Check sheet for the drawn part. Datum: minimum x, y, z corner. Units: mm. A direction names the side the tool comes from. Give positions to 0.01 mm unless a question says otherwise; leave off trailing zeros. Order: outer loops, then holes, each group sorted by start corner. A loop starts at its lowest first (then second) coordinate and runs counter-clockwise, first axis right, second up. Notation, with made-up numbers: (88, 51) - (96, 51) arc R24 cw to (96, 62) - close; hole circle Ø7 at (-12, 77.25). An arc over 180 degrees is marked (long way). Answer as a JSON object with one key per item and string values. Group by question number.
(1) Section check D-D (y = 15). Record the boundary of the cut face in (x, z).
(2) Section check C-C (z = 12). Record the boundary of the cut face in (x, y), then the cut area to 3 significant figures.
(3) Access from +Z, -Z, +X, -X, +Y, -Y to the whole of each face (thin tool, end or side, straight path). Record for the marked faces 5 and 6.
(4) Section check A-A (x = 21). Record the boundary of the cut face in (y, z).
(5) Depth check by flat-ended pin: pin 1 Ø6 at (x, z) = (27.5, 10.5) entering from +Y; pin 2 Ø1 at (x, z) = (18, 16.5) entering from -Y; pin 3 Ø13 at (x, y) = (18.5, 22.5) entering from -Z; pin 4 Ø10 at (x, z) = (20.5, 25) entering from -Y. Enter the tip coordinate at first touch or a pass-through.
(6) Mould release check, pull along Z, two halves, no side actions. Record for the marked faces 1, 2, 3 and 4: +Z half, -Z half, draft (parallel to the pull), parting line (faces both ways), or undercut.
(7) Section check B-B (z = 32). Record the boundary of the cut face in (x, y), then the cut area to 3 significant figures.
(8) Thickness scan on line 1 (Y direction, x = 29, z = 33.5); line 2 (X direction, y = 32.5, z = 8); line 3 (Y direction, x = 13, z = 31) (3 decimals). Record the ranges inside material, lowest first.
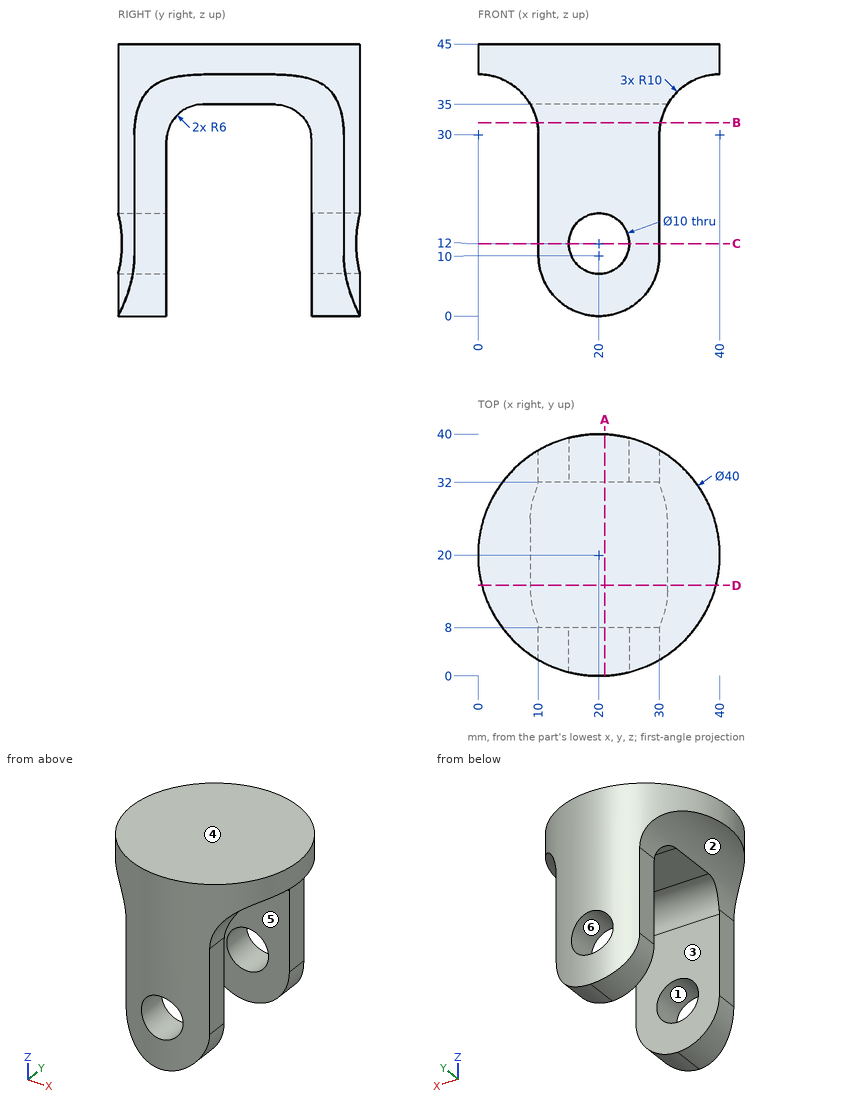
Solutions:
{
 "1": {"outline": "(0.64, 39.98) arc R10 cw to (8.66, 35) - (31.34, 35) arc R10 cw to (39.36, 39.98) - (39.36, 45) - (0.64, 45) - close"},
 "2": {"outline": "(10, 2.68) arc R20 ccw to (15, 0.64) - (15, 8) - (10, 8) - close; (10, 32) - (15, 32) - (15, 39.36) arc R20 ccw to (10, 37.32) - close; (25, 0.64) arc R20 ccw to (30, 2.68) - (30, 8) - (25, 8) - close; (25, 32) - (30, 32) - (30, 37.32) arc R20 ccw to (25, 39.36) - close", "area": "129 mm2"},
 "3": {"face 5": "-Z, +X, -X", "face 6": "+Y, -Y"},
 "4": {"outline": "(0.03, 0.05) - (8, 0.05) - (8, 7.1) - (0.03, 7.1) - close; (0.03, 16.9) - (8, 16.9) - (8, 29) arc R6 cw to (14, 35) - (26, 35) arc R6 cw to (32, 29) - (32, 16.9) - (39.97, 16.9) - (39.97, 45) - (0.03, 45) - close; (32, 0.05) - (39.97, 0.05) - (39.97, 7.1) - (32, 7.1) - close"},
 "5": {"pin 1": "stops at y = 39.47", "pin 2": "stops at y = 0.06", "pin 3": "stops at z = 34.2", "pin 4": "stops at y = 0"},
 "6": {"face 1": "undercut", "face 2": "-Z half", "face 3": "draft", "face 4": "+Z half"},
 "7": {"outline": "(9.8, 2.8) arc R20 ccw to (30.2, 2.8) - (30.2, 8.8) - (9.8, 8.8) - close; (9.8, 31.2) - (30.2, 31.2) - (30.2, 37.2) arc R20 ccw to (9.8, 37.2) - close", "area": "322 mm2"},
 "8": {"line 1": "y = 2.14 to 10.03, 29.97 to 37.86", "line 2": "x = 10.2 to 17, 23 to 29.8", "line 3": "y = 1.265 to 8.343, 31.657 to 38.735"}
}
